Read the model definition and answer for the solid it produces. Units are mm, in the model's axes. Round coordinates to 2 decimals unless told otherwise and drop trailing zeros. Loops run counter-clockwise (first coordinate to the right, second up) from the corner with the lowest first, then second, coordinate; pieces in that order, holes last. Notation, with made-up numbers: (-16.5, -20) -> (21.5, -20) arc R28 cw to (21.5, 0) -> close; hole circle Ø3 at (70, 0). An arc over 180 degrees is marked (long way). Put each result on its own line as item: value.
from build123d import *

# Parameters (mm, degrees)
BOSS_EXTRUDE1_DEPTH     = 1726.350547376
SKETCH2_W               = 211.702458594
SKETCH2_H               = 483.586926944
CUT_EXTRUDE1_DEPTH      = 34.517974046
SKETCH3_W               = 200.611820877
SKETCH3_H               = 857.421683483
CUT_EXTRUDE3_DEPTH      = 93.089876837
CUT_EXTRUDE3_DEPTH_BACK = 2.54


with BuildPart() as part:
    # Sketch1 → Boss-Extrude1 (new body)
    with BuildSketch(Plane.XY):
        with BuildLine():
            Line((-27.5, 49), (27.5, 49))
            Line((27.5, 49), (27.5, 44.3))
            Line((27.5, 44.3), (8.8, 44.3))
            ThreePointArc((8.8, 44.3), (3.850252532, 42.249747468), (1.8, 37.3))
            Line((1.8, 37.3), (1.8, -37.3))
            ThreePointArc((1.8, -37.3), (3.850252532, -42.249747468), (8.8, -44.3))
            Line((8.8, -44.3), (27.5, -44.3))
            Line((27.5, -44.3), (27.5, -49))
            Line((27.5, -49), (-27.5, -49))
            Line((-27.5, -49), (-27.5, -44.3))
            Line((-27.5, -44.3), (-8.8, -44.3))
            ThreePointArc((-8.8, -44.3), (-3.850252532, -42.249747468), (-1.8, -37.3))
            Line((-1.8, -37.3), (-1.8, 37.3))
            ThreePointArc((-1.8, 37.3), (-3.850252532, 42.249747468), (-8.8, 44.3))
            Line((-8.8, 44.3), (-27.5, 44.3))
            Line((-27.5, 44.3), (-27.5, 49))
        make_face()
    extrude(amount=BOSS_EXTRUDE1_DEPTH)

    # Sketch2 → Cut-Extrude1 (cut, through all)
    with BuildSketch(Plane(origin=(0, -5.731911144, 15.748296437), x_dir=(1, 0, 0), z_dir=(0, -0.342020143, 0.939692621))):
        with Locations((0, 13.030857736)):
            Rectangle(SKETCH2_W, SKETCH2_H)
    extrude(amount=-CUT_EXTRUDE1_DEPTH, mode=Mode.SUBTRACT)

    # Sketch3 → Cut-Extrude3 (cut, two sides)
    with BuildSketch(Plane(origin=(0, 511.570282058, 186.196355404), x_dir=(1, 0, 0), z_dir=(0, 0.939692621, 0.342020143))) as cut_extrude3_sk:
        with Locations((34.7211676, -1334.740482361)):
            Rectangle(SKETCH3_W, SKETCH3_H)
    extrude(amount=CUT_EXTRUDE3_DEPTH, mode=Mode.SUBTRACT)
    extrude(cut_extrude3_sk.sketch, amount=-CUT_EXTRUDE3_DEPTH_BACK, mode=Mode.SUBTRACT)


solid = part.part
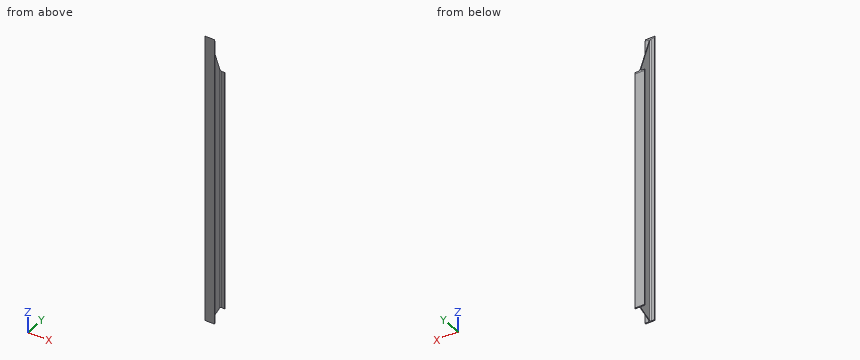
Item 1: The part is cut by section A-A (z = 259). Determine the outline of the cut face in (x, y).
Derived:
outline: (-27.5, -49) -> (27.5, -49) -> (27.5, -44.3) -> (8.8, -44.3) arc R7 cw to (1.8, -37.3) -> (1.8, 37.3) arc R7 cw to (8.8, 44.3) -> (27.5, 44.3) -> (27.5, 49) -> (-27.5, 49) -> (-27.5, 44.3) -> (-8.8, 44.3) arc R7 cw to (-1.8, 37.3) -> (-1.8, -37.3) arc R7 cw to (-8.8, -44.3) -> (-27.5, -44.3) -> close
Item 2: Find the intervals of material crossed by line 1 along Y through (x, z) = (-25, 1413.5); line 2 along X through (y, z) = (-23, 719); line 3 along X through (y, z) = (-39, 1410), in increasing order.
Derived:
line 1: y = -49 to -44.3, 44.3 to 49
line 2: x = -1.8 to 1.8
line 3: x = -2.01 to 2.01
Item 3: The part is cut by section B-B (y = 15.5). Determine the outline of the cut face in (x, z).
Derived:
outline: (-1.8, 23.48) -> (1.8, 23.48) -> (1.8, 1541.71) -> (-1.8, 1541.71) -> close
Item 4: Flat-ended cylindrical pins translate along their axes: pin 1 Ø1.5 at (y, z) = (8.5, 502.5) entering from -X; pin 2 Ø8 at (y, z) = (9.5, 1215.5) entering from +X; pin 3 Ø12 at (x, y) = (3, -39) entering from -Z. Find the tip coordinate at first contact, or state that the pin passes through.
Derived:
pin 1: stops at x = -1.8
pin 2: stops at x = 1.8
pin 3: stops at z = 1.46
Item 5: The part is cut by section C-C (z = 1505). Determine the outline of the cut face in (x, y).
Derived:
outline: (-27.5, -49) -> (27.5, -49) -> (27.5, -44.3) -> (8.8, -44.3) arc R7 cw to (1.8, -37.3) -> (1.8, 28.86) -> (-1.8, 28.86) -> (-1.8, -37.3) arc R7 cw to (-8.8, -44.3) -> (-27.5, -44.3) -> close
